```python
from build123d import *

# Parameters (mm, degrees)
F0_R     = 4
F1_DEPTH = 8
F2_R     = 2
F3_DEPTH = 5
F5_DEPTH = 3


with BuildPart() as f1:
    # F0 (on Top) → F1 (new body)
    with BuildSketch(Plane.XY):
        with BuildLine():
            Line((20, 0), (0, 0))
            Line((0, 0), (0, -60))
            Line((0, -60), (10, -60))
            ThreePointArc((10, -60), (17.0710678119, -57.0710678119), (20, -50))
            Line((20, -50), (20, 0))
        make_face()
        with Locations((10, -50)):
            Circle(F0_R, mode=Mode.SUBTRACT)
        with BuildLine():
            Line((0, -60), (0, 0))
            Line((0, 0), (-20, 0))
            Line((-20, 0), (-20, -50))
            ThreePointArc((-20, -50), (-17.0710678119, -57.0710678119), (-10, -60))
            Line((-10, -60), (0, -60))
        make_face()
        with Locations((-10, -50)):
            Circle(F0_R, mode=Mode.SUBTRACT)
    extrude(amount=F1_DEPTH)

    # F2 (on Front) → F3 (join)
    with BuildSketch(Plane.XZ):
        Polygon((-3, 8), (3, 8), (3, 28), (0, 28), (-3, 28), align=None)
        with BuildLine():
            Line((3, 8), (20, 8))
            Line((20, 8), (30.1036297108, 25.5))
            ThreePointArc((30.1036297108, 25.5), (30.1036297108, 30.5), (25.7735026919, 33))
            Line((25.7735026919, 33), (0, 33))
            Line((0, 33), (-25.7735026919, 33))
            ThreePointArc((-25.7735026919, 33), (-30.1036297108, 30.5), (-30.1036297108, 25.5))
            Line((-30.1036297108, 25.5), (-20, 8))
            Line((-20, 8), (-3, 8))
            Line((-3, 8), (-3, 28))
            Line((-3, 28), (0, 28))
            Line((0, 28), (3, 28))
            Line((3, 28), (3, 8))
        make_face()
        with BuildLine():
            Line((-20.77, 28), (-8, 28))
            Line((-8, 28), (-8, 13))
            Line((-8, 13), (-17.1132486541, 13))
            Line((-17.1132486541, 13), (-23.272627479, 23.6683570679))
            ThreePointArc((-23.272627479, 23.6683570679), (-21.4406315354, 25.4986866055), (-20.77, 28))
        make_face(mode=Mode.SUBTRACT)
        with Locations((-25.77, 28)):
            Circle(F2_R, mode=Mode.SUBTRACT)
        with BuildLine():
            Line((8, 13), (8, 28))
            Line((8, 28), (20.77, 28))
            ThreePointArc((20.77, 28), (21.4406315354, 25.4986866055), (23.272627479, 23.6683570679))
            Line((23.272627479, 23.6683570679), (17.1132486541, 13))
            Line((17.1132486541, 13), (8, 13))
        make_face(mode=Mode.SUBTRACT)
        with Locations((25.77, 28)):
            Circle(F2_R, mode=Mode.SUBTRACT)
    extrude(amount=F3_DEPTH)

    # F4 (on Right) → F5 (join, symmetric)
    with BuildSketch(Plane.YZ):
        Polygon((-50, 8), (-5, 8), (-5, 25.5), (-5, 28.0183628846), (-60, 8), align=None)
        Polygon((-31.6435909019, 13), (-10, 20.8776228509), (-10, 13), align=None, mode=Mode.SUBTRACT)
    extrude(amount=F5_DEPTH, both=True)


solid = f1.part
```
Model file for the job. Use its own axes, mm. A direction names the side the tool comes from. Coordinates: 2 decimals unless noted, no trailing zeros. Loops run counter-clockwise (first coordinate to the right, second up) from the corner with the lowest first, then second, coordinate; pieces in that order, holes last. Notation, with made-up numbers: (20.5, 57) - (73.5, 57) arc R19 cw to (73.5, 74) - close; hole circle Ø9 at (-12, 18). An arc over 180 degrees is marked (long way). Answer as a JSON object with one key per item and string values. Group by question number.
(1) Probe line 1 along Y through (x, z) = (10, 3); line 2 along X through (y, z) = (-50.5, 1.5); line 3 along Z through (x, y) = (19, -49). List the from-to ranges inside material, lowest first.
(2) Cut at B-B (y = -53). Give the cut face in (x, z), then the cut area to 3 significant figures.
(3) Two-plate mould, pull along Y, no slides. Class faces 1 (the face through (0.042, -32.115, 18.149)), 2 (the face through (6.8, -52.4, 3.9)), 3 (the face through (-20, -2, 18)): released by +Y, released by -Y, zero draft, split by the parting line, or undercut.
(4) Tool access for faces 4 (the face through (-8, -2, 21)), 5 (the face through (-12, -32, 8)), 6 (the face through (0.042, -20.973, 16.884)), 7 (the face through (0, -2, 33)), 8 (the face through (-17.15, -56.99, 3.94)): list every direction of +Z, -Z, +X, -X, +Y, -Y with a clear straight run to the whole face (end or side of a thin tool).
(5) Flat gauge pins, fed straight in: pin 1 (6.5 mm diameter, centred on x = 10, y = -50, fed in from -Z); pin 2 (18.5 mm diameter, centred on x = -14, y = -22, fed in from +Z); pin 3 (8 mm diameter, centred on y = -34.5, z = 11, fed in from +X); pin 4 (1.8 mm diameter, centred on x = 0.5, y = -19, fed in from +Z). Where does each tip first touch, or does it go through?
(6) Cut at C-C (x = -22). Give the cut face in (y, z), then the cut area to 3 significant figures.
(7) Cut at D-D (x = 9). Give the cut face in (y, z).
(8) Cut at A-A (z = 6.5). Give the cut face in (x, y).
Geometry says:
{
 "1": {"line 1": "y = -60 to -54, -46 to 0", "line 2": "x = -19.99 to -13.97, -6.03 to 6.03, 13.97 to 19.99", "line 3": "z = 0 to 8"},
 "2": {"outline": "(-19.54, 0) - (-12.65, 0) - (-12.65, 8) - (-19.54, 8) - close; (-7.35, 0) - (7.35, 0) - (7.35, 8) - (3, 8) - (3, 10.55) - (-3, 10.55) - (-3, 8) - (-7.35, 8) - close; (12.65, 0) - (19.54, 0) - (19.54, 8) - (12.65, 8) - close", "area": "243 mm^2"},
 "3": {"face 1": "released by -Y", "face 2": "undercut", "face 3": "zero draft"},
 "4": {"face 4": "+Y, -Y", "face 5": "+Z, -X, -Y", "face 6": "+X, -X", "face 7": "+Z, +X, -X, +Y, -Y", "face 8": "+Z, -Z, -X, -Y"},
 "5": {"pin 1": "passes through", "pin 2": "stops at z = 8", "pin 3": "stops at x = 20", "pin 4": "stops at z = 23.25"},
 "6": {"outline": "(-5, 11.46) - (0, 11.46) - (0, 21.46) - (-5, 21.46) - close; (-5, 24.72) - (0, 24.72) - (0, 33) - (-5, 33) - close", "area": "91.4 mm^2"},
 "7": {"outline": "(-60, 0) - (-53.87, 0) - (-53.87, 8) - (-60, 8) - close; (-46.13, 0) - (0, 0) - (0, 13) - (-5, 13) - (-5, 8) - (-46.13, 8) - close; (-5, 28) - (0, 28) - (0, 33) - (-5, 33) - close"},
 "8": {"outline": "(-20, -50) arc R10 ccw to (-10, -60) - (10, -60) arc R10 ccw to (20, -50) - (20, 0) - (-20, 0) - close; hole circle Ø8 at (-10, -50); hole circle Ø8 at (10, -50)"}
}
